Read the model definition and answer for the solid it produces. Units are mm, in the model's axes. Face numbers are marked on the shaded views. Coordinates: 2 decimals unless noted, no trailing zeros. Order: outer loops, then holes, each group sorted by start corner. A loop starts at its lowest first (then second) coordinate and runs counter-clockwise, first axis right, second up.
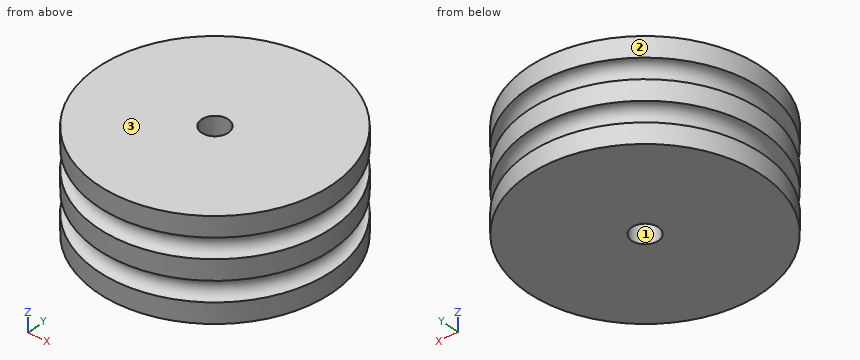
from build123d import *

# Parameters (mm, degrees)
TORUS001_R     = 1.5
TORUS_R        = 1.5
CYLINDER_R     = 17.5
CYLINDER_DEPTH = 15
SKETCH_R       = 2
POCKET_DEPTH   = 15.001


with BuildPart() as bottom_o_ring:
    # Torus001 → Torus001 (revolve)
    with BuildSketch(Plane(origin=(0, 0, 4.5), x_dir=(1, 0, 0), z_dir=(0, -1, 0))):
        with Locations((17.5, 0)):
            Circle(TORUS001_R)
    revolve(axis=Axis((0, 0, 4.5), (0, 0, 1)))


with BuildPart() as o_rings:
    # Torus → Torus (revolve)
    with BuildSketch(Plane(origin=(0, 0, 10.5), x_dir=(1, 0, 0), z_dir=(0, -1, 0))):
        with Locations((17.5, 0)):
            Circle(TORUS_R)
    revolve(axis=Axis((0, 0, 10.5), (0, 0, 1)))

    # Fusion: union bottom-o-ring
    add(bottom_o_ring.part)


with BuildPart() as drill_axle:
    # Cylinder → Cylinder (new body)
    with BuildSketch(Plane.XY):
        Circle(CYLINDER_R)
    extrude(amount=CYLINDER_DEPTH)

    # Cut: cut o-rings
    add(o_rings.part, mode=Mode.SUBTRACT)

    # Sketch → Pocket (cut, through all)
    with BuildSketch(Plane.XY.offset(15)):
        Circle(SKETCH_R)
    extrude(amount=-POCKET_DEPTH, mode=Mode.SUBTRACT)


solid = drill_axle.part
Q1. The part is cut by section A-A, the plane x = 0. Determine the outline of the cut face in (y, z), then the cut area to 3 significant figures.
Q2. Each of these flat-tipped pins is pushed along its axis until it touches: P1, Ø8, axis at x = -11.5, z = 1.5, coming from the -Y side; P2, Ø6, axis at x = -8, z = 4.5, coming from the +Y side; P3, Ø3, axis at x = 0, y = 0, coming from the -Z side; P4, Ø3, axis at y = -7, z = 3, coming from the -X side. Where does it stop, or does it pass through?
Q3. The part is cut by section C-C, the plane z = 3.5. Determine the outline of the cut face in (x, y), then the cut area to 3 significant figures.
Q4. Determine the mould class of the marked faces 1, 2 and 3 for opening direction X: +X half, -X half, draft (parallel to the pull), parting line (faces both ways), or undercut.
Q5. Straight lines are drawn through the part: L1, parallel to Z at x = 10, y = 14; L2, parallel to Y at x = 0, z = 10.25; L3, parallel to Y at x = 0, z = 5.5. For each, find the intervals that lie inside material, in ascending order.
Computed values:
1. outline: (-17.5, 0) - (-2, 0) - (-2, 15) - (-17.5, 15) - (-17.5, 12) arc R1.5 cw to (-17.5, 9) - (-17.5, 6) arc R1.5 cw to (-17.5, 3) - close; (2, 0) - (17.5, 0) - (17.5, 3) arc R1.5 cw to (17.5, 6) - (17.5, 9) arc R1.5 cw to (17.5, 12) - (17.5, 15) - (2, 15) - close
1. area: 451 mm2
2. P1: stops at y = -15.81
2. P2: stops at y = 16.65
2. P3: passes through
2. P4: stops at x = -16.61
3. outline: circle Ø32.76 at (0, 0); hole circle Ø4 at (0, 0)
3. area: 831 mm2
4. face 1: undercut
4. face 2: parting line
4. face 3: draft
5. L1: z = 0 to 3.03, 5.97 to 9.03, 11.97 to 15
5. L2: y = -16.02 to -2, 2 to 16.02
5. L3: y = -16.38 to -2, 2 to 16.38
